Check sheet for the modelled part. Datum: model origin and axes. Units: mm. Round coordinates to 2 decimals unless told otherwise and drop trailing zeros. Order: outer loops, then holes, each group sorted by start corner. A loop starts at its lowest first (then second) coordinate and runs counter-clockwise, first axis right, second up.
```python
from build123d import *

# Parameters (mm, degrees)
SKETCH1_W            = 152.4
SKETCH1_H            = 34.925
MASS_DEPTH           = 6.35
SKETCH3_W            = 12.7
SKETCH3_H            = 12.7
TOP_TOOTH_DEPTH      = 6.35
TOP_PUZZLE_COUNT     = 3
TOP_PUZZLE_PITCH     = 25.4
TOP_PUZZLE_COL_COUNT = 3
TOP_PUZZLE_COL_PITCH = 25.4
SKETCH4_W            = 12.7
SKETCH4_H            = 12.7
SIDE_TOOTH_DEPTH     = 81.086188923


with BuildPart() as part:
    # Sketch1 → Mass (new body)
    with BuildSketch(Plane.XY):
        Rectangle(SKETCH1_W, SKETCH1_H)
    extrude(amount=MASS_DEPTH)

    # Sketch3 → Top Tooth (add)
    with BuildSketch(Plane(origin=(0, 0, 0), x_dir=(-1, 0, 0), z_dir=(0, 0, -1))):
        with Locations((0, 17.4625)):
            Rectangle(SKETCH3_W, SKETCH3_H)
        with Locations((0, -17.4625)):
            Rectangle(SKETCH3_W, SKETCH3_H)
    top_tooth = extrude(amount=-TOP_TOOTH_DEPTH)

    # Top Puzzle: Top Tooth ×3
    with Locations(*[(-i * TOP_PUZZLE_PITCH, 0, 0) for i in range(1, TOP_PUZZLE_COUNT)]):
        add(top_tooth)

    # Top Puzzle col: Top Tooth ×3
    with Locations(*[(i * TOP_PUZZLE_COL_PITCH, 0, 0) for i in range(1, TOP_PUZZLE_COL_COUNT)]):
        add(top_tooth)

    # Sketch4 → Side Tooth (cut, through all)
    with BuildSketch(Plane.XY.offset(6.35)):
        with Locations((76.2, 0)):
            Rectangle(SKETCH4_W, SKETCH4_H)
        with Locations((-76.2, 0)):
            Rectangle(SKETCH4_W, SKETCH4_H)
    extrude(amount=-SIDE_TOOTH_DEPTH, mode=Mode.SUBTRACT)


solid = part.part
```
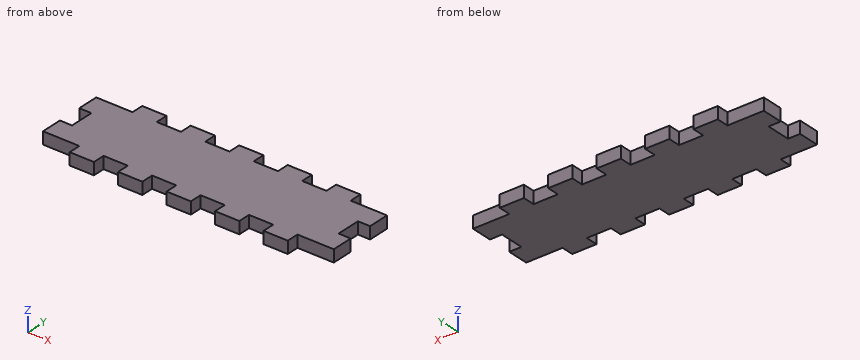
Item 1: Go/stop test with flat-tipped pins: P1, Ø3, axis at y = 22, z = 2, coming from the +X side; P2, Ø3, axis at x = -39.5, z = 3, coming from the -Y side; P3, Ø1.9, axis at x = 72.5, z = 4, coming from the +Y side. Record where each tip stops, or that it passes through.
Answer:
P1: stops at x = 57.15
P2: stops at y = -17.46
P3: stops at y = 17.46
Item 2: Sectioned sample at B-B (y = -1.5). Record the cut outline in (x, z), and give its area (3 significant figures).
Answer:
outline: (-69.85, 0) - (69.85, 0) - (69.85, 6.35) - (-69.85, 6.35) - close
area: 887 mm2
Item 3: Scan lines: line 1 along X through (y, z) = (-19, 1); line 2 along X through (y, z) = (6, 0.5); line 3 along Y through (x, z) = (66, 5.75). Record each from-to range of solid material in increasing order.
Answer:
line 1: x = -57.15 to -44.45, -31.75 to -19.05, -6.35 to 6.35, 19.05 to 31.75, 44.45 to 57.15
line 2: x = -69.85 to 69.85
line 3: y = -17.46 to 17.46
Item 4: Sectioned sample at A-A (x = -36). Record the cut outline in (y, z).
Answer:
outline: (-17.46, 0) - (17.46, 0) - (17.46, 6.35) - (-17.46, 6.35) - close
